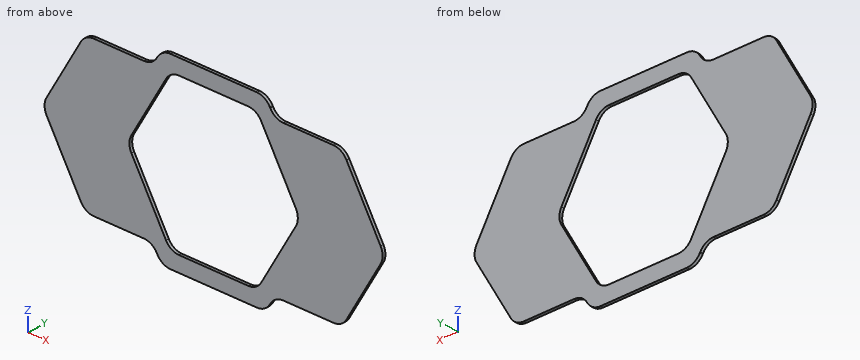
```python
from build123d import *

# Parameters (mm, degrees)
F1_DEPTH = 5.08
F2_R     = 25.4


with BuildPart() as f1:
    # F0 (on Front) → F1 (new body)
    with BuildSketch(Plane.XZ):
        Polygon((-72.5902493452, -125.73), (41.7943859866, -125.73), (-30.7958633586, 0), (41.7943859866, 125.73), (-72.5902493452, 125.73), (-145.1804986904, 0), align=None)
        Polygon((41.7943859866, -125.73), (71.1237796615, -125.73), (-1.4664696837, 0), (71.1237796615, 125.73), (41.7943859866, 125.73), (-30.7958633586, 0), align=None)
        Polygon((41.7943859866, 125.73), (71.1237796615, 125.73), (71.8570145033, 127), (218.5039828775, 127), (219.2372177194, 125.73), (248.5666113942, 125.73), (233.1686797149, 152.4), (57.1923176659, 152.4), align=None)
        Polygon((291.8274670646, 0), (219.2372177194, -125.73), (248.5666113942, -125.73), (321.1568607394, 0), (248.5666113942, 125.73), (219.2372177194, 125.73), align=None)
        Polygon((321.1568607394, 0), (248.5666113942, -125.73), (362.9512467261, -125.73), (435.5414960713, 0), (362.9512467261, 125.73), (248.5666113942, 125.73), align=None)
        Polygon((71.8570145033, -127), (71.1237796615, -125.73), (41.7943859866, -125.73), (57.1923176659, -152.4), (233.1686797149, -152.4), (248.5666113942, -125.73), (219.2372177194, -125.73), (218.5039828775, -127), align=None)
    extrude(amount=F1_DEPTH)

    # F2
    f2_edges = [f1.edges().sort_by_distance(p)[0] for p in [
        (41.794386, -2.54, 125.73),
        (-72.590249, -2.54, 125.73),
        (-145.180499, -2.54, 0),
        (-72.590249, -2.54, -125.73),
        (41.794386, -2.54, -125.73),
        (57.192318, -2.54, -152.4),
        (233.16868, -2.54, -152.4),
        (248.566611, -2.54, -125.73),
        (362.951247, -2.54, -125.73),
        (435.541496, -2.54, 0),
        (362.951247, -2.54, 125.73),
        (248.566611, -2.54, 125.73),
        (233.16868, -2.54, 152.4),
        (57.192318, -2.54, 152.4),
        (71.857015, -2.54, 127),
        (218.503983, -2.54, 127),
        (291.827467, -2.54, 0),
        (218.503983, -2.54, -127),
        (71.857015, -2.54, -127),
        (-1.46647, -2.54, 0),
    ]]
    fillet(f2_edges, radius=F2_R)


solid = f1.part
```
Geometry check sheet. Reference: the model listing, model coordinates, mm. Coordinates: 2 decimals unless noted, no trailing zeros. Order: outer loops, then holes, each group sorted by start corner. A loop starts at its lowest first (then second) coordinate and runs counter-clockwise, first axis right, second up. Notation, with made-up numbers: (-11, 16) - (7, 16) arc R23 ccw to (7, 50) - close; hole circle Ø8 at (4.5, 50.25). An arc over 180 degrees is marked (long way). Answer in a Markdown table with one row per item. Add a question column.
1. Material ranges on L1, parallel to Z at x = 184, y = -2.4; L2, parallel to X at y = -1.75, z = 1.5; L3, parallel to Z at x = -1.5, y = -1.6, recorded low to high. Write a range as [from, to].
2. Section check B-B (z = 64). Enter the section's corners in (x, y), plus the area to 3 significant figures.
3. Gauge pin test, flat ends, axial feed: pin 1 Ø1 at (x, z) = (-80.5, -52.5) entering from +Y; pin 2 Ø2.5 at (x, y) = (305, -3) entering from -Z. Record the tip position at first contact, or that the pin passes through.
4. Section check A-A (x = 198). Enter the section's corners in (y, z), plus the area to 3 significant figures.
Data:
| question | item | result |
|---|---|---|
| 1 | L1 | z = [-152.4, -127], [127, 152.4] |
| 1 | L2 | x = [-141.21, 2.51], [287.85, 431.57] |
| 1 | L3 | z = [-125.73, 125.73] |
| 2 | outline | (-108.23, -5.08) - (35.48, -5.08) - (35.48, 0) - (-108.23, 0) - close; (254.88, -5.08) - (398.59, -5.08) - (398.59, 0) - (254.88, 0) - close |
| 2 | area | 1,460 mm² |
| 3 | pin 1 | stops at y = 0 |
| 3 | pin 2 | stops at z = -125.73 |
| 4 | outline | (-5.08, -152.4) - (0, -152.4) - (0, -127) - (-5.08, -127) - close; (-5.08, 127) - (0, 127) - (0, 152.4) - (-5.08, 152.4) - close |
| 4 | area | 258 mm² |
